Input: part model. Units: mm. Frame: model coordinates. Face numbers are marked on the shaded views. A direction names the side the tool comes from. Round coordinates to 2 decimals unless told otherwise and drop trailing zeros. Loops run counter-clockwise (first coordinate to the right, second up) from the corner with the lowest first, then second, coordinate; pieces in that order, holes last. Notation, with made-up numbers: M -11.75,63.25 L 7.25,63.25 A4 cw 7.25,67.25 Z; hole C -39.5,67.5 d10. An arc over 180 degrees is marked long. Put each result on its own line as item: value. Start each with the question number.
1) Section A-A on x = 180. Output: boundary loops of the cut face in (y, z).
2) Section C-C on y = 83. Output: boundary loops of the cut face in (x, z), plus the area to 3 significant figures.
3) Line query: probe 1 along Y at (x, z) = (90, 39); probe 2 along X at (y, z) = (17, 0); probe 3 along Z at (x, y) = (133, 128). Output: solid intervals per line, ascending.
4) Reachability of the marked faces 1, 2 and 3 from +Z, -Z, +X, -X, +Y, -Y: full face, straight path, thin tool, end or side. Return the list, or none.
5) Section B-B on z = 0. Output: boundary loops of the cut face in (x, y), plus the area to 3 significant figures.
6) Pin query (flat end, axial travel): pin 1 (20 mm diameter, centred on x = 90, y = 100, fed in from -Z); pin 2 (4 mm diameter, centred on x = 162, z = 7, fed in from +Y); pin 3 (24 mm diameter, centred on x = 107, y = 63.5, fed in from +Z); pin 4 (4 mm diameter, centred on y = 126.5, z = -14.5, fed in from -X). Return the tip coordinate at first contact, or that it passes through.
7) Draft query along X for the marked faces 4, 5 and 6. Return one class per face: +X half, -X half, draft (parallel to the pull), parting line (faces both ways), or undercut.
8) Section D-D on z = 45.5. Output: boundary loops of the cut face in (x, y).
from build123d import *

# Parameters (mm, degrees)
BOSS_EXTRUDE1_DEPTH = 50
FILLET1_R           = 30
SKETCH2_R           = 50
BOSS_EXTRUDE2_DEPTH = 60
SKETCH3_R           = 30
CUT_EXTRUDE1_DEPTH  = 121
FILLET2_R           = 10
CUT_EXTRUDE2_DEPTH  = 25
SKETCH6_R           = 12.5
CUT_EXTRUDE3_DEPTH  = 111
FILLET3_R           = 25
SKETCH10_R          = 12.5
CUT_EXTRUDE5_DEPTH  = 31


with BuildPart() as part:
    # Sketch1 → Boss-Extrude1 (new body, symmetric)
    with BuildSketch(Plane.XY):
        Polygon((0, 0), (290, 0), (290, 30), (230, 30), (230, 130), (60, 130), (60, 30), (0, 30), align=None)
    extrude(amount=BOSS_EXTRUDE1_DEPTH, both=True)

    # Fillet1
    fillet1_edges = [part.edges().sort_by_distance(p)[0] for p in [
        (60, 130, 0),
        (230, 130, 0),
    ]]
    fillet(fillet1_edges, radius=FILLET1_R)

    # Sketch2 → Boss-Extrude2 (add, symmetric)
    with BuildSketch(Plane.XY):
        with Locations((180, 100)):
            Circle(SKETCH2_R)
    extrude(amount=BOSS_EXTRUDE2_DEPTH, both=True)

    # Sketch3 → Cut-Extrude1 (cut, through all)
    with BuildSketch(Plane.XY.offset(60)):
        with Locations((180, 100)):
            Circle(SKETCH3_R)
    extrude(amount=-CUT_EXTRUDE1_DEPTH, mode=Mode.SUBTRACT)

    # Fillet2
    fillet2_edges = [part.edges().sort_by_distance(p)[0] for p in [
        (60, 30, 0),
        (230, 30, 0),
    ]]
    fillet(fillet2_edges, radius=FILLET2_R)

    # Sketch5 → Cut-Extrude2 (cut, symmetric)
    with BuildSketch(Plane.XY):
        with BuildLine():
            Line((140, 130), (60, 130))
            Line((60, 130), (60, 40))
            Line((60, 40), (130, 40))
            Line((130, 40), (130, 100))
            ThreePointArc((130, 100), (132.565835097, 115.811388301), (140, 130))
        make_face()
    extrude(amount=CUT_EXTRUDE2_DEPTH, both=True, mode=Mode.SUBTRACT)

    # Sketch6 → Cut-Extrude3 (cut, through all)
    with BuildSketch(Plane.XY.offset(50)):
        with Locations((90, 100)):
            Circle(SKETCH6_R)
        with Locations((90, 58)):
            Circle(SKETCH6_R)
    extrude(amount=-CUT_EXTRUDE3_DEPTH, mode=Mode.SUBTRACT)

    # Fillet3
    fillet3_edges = [part.edges().sort_by_distance(p)[0] for p in [
        (290, 15, 50),
        (0, 15, -50),
        (0, 15, 50),
        (290, 15, -50),
    ]]
    fillet(fillet3_edges, radius=FILLET3_R)

    # Sketch10 → Cut-Extrude5 (cut, through all)
    with BuildSketch(Plane(origin=(0, 30, 0), x_dir=(1, 0, 0), z_dir=(0, 1, 0))):
        with Locations(Location((30, 0, 0), (0, 0, 270))):  # turned: the seam where the file's is
            Circle(SKETCH10_R)
        with Locations(Location((260, 0, 0), (0, 0, 270))):  # turned: the seam where the file's is
            Circle(SKETCH10_R)
    extrude(amount=-CUT_EXTRUDE5_DEPTH, mode=Mode.SUBTRACT)


solid = part.part
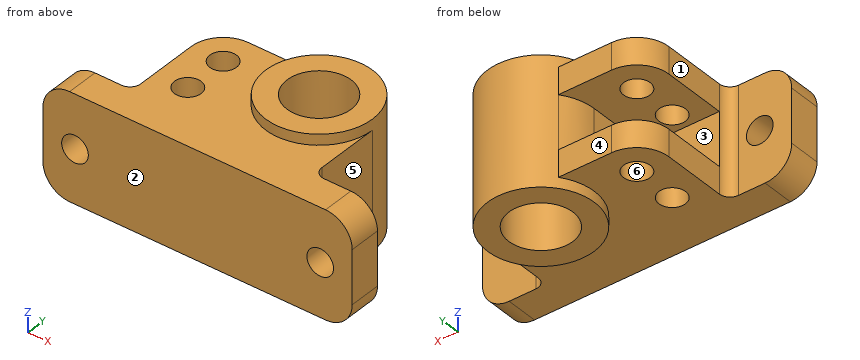
Geometry results:
1. outline: M 0,-50 L 50,-50 L 50,-60 L 70,-60 L 70,60 L 50,60 L 50,50 L 0,50 Z; M 130,-60 L 150,-60 L 150,60 L 130,60 Z
2. outline: M 60,-50 L 132.98,-50 L 132.98,-60 L 155.28,-60 L 155.28,60 L 132.98,60 L 132.98,50 L 60,50 L 60,25 L 130,25 L 130,-25 L 60,-25 Z; M 204.72,-60 L 227.02,-60 L 227.02,-50 L 230,-50 L 230,50 L 227.02,50 L 227.02,60 L 204.72,60 Z
2. area: 9,450 mm²
3. probe 1: y = 0 to 45.5, 70.5 to 87.5, 112.5 to 130
3. probe 2: x = 0 to 17.5, 42.5 to 247.5, 272.5 to 290
3. probe 3: z = -50 to -25, 25 to 50
4. face 1: +Z, -Z, -X, +Y
4. face 2: +Z, -Z, +X, -X, -Y
4. face 3: -X, +Y
5. outline: M 0,0 L 17.5,0 L 17.5,30 L 0,30 Z; M 42.5,0 L 247.5,0 L 247.5,30 L 240,30 A10 cw 230,40 L 230,100 A50 ccw 130,100 L 130,40 L 60,40 A10 cw 50,30 L 42.5,30 Z; M 272.5,0 L 290,0 L 290,30 L 272.5,30 Z; hole C 180,100 d60
5. area: 16,000 mm²
6. pin 1: passes through
6. pin 2: stops at y = 147.37
6. pin 3: stops at z = 50
6. pin 4: stops at x = 136.41
7. face 4: draft
7. face 5: +X half
7. face 6: undercut
8. outline: M 10.69,0 L 279.31,0 L 279.31,30 L 240,30 A10 cw 230,40 L 230,100 A50 ccw 140,130 L 90,130 A30 ccw 60,100 L 60,40 A10 cw 50,30 L 10.69,30 Z; hole C 90,58 d25; hole C 90,100 d25; hole C 180,100 d60
